Check sheet for the modelled part. Datum: model origin and axes. Units: mm. A direction names the side the tool comes from. Give positions to 0.01 mm unless a question says otherwise; leave off trailing zeros. Write each loop counter-clockwise with the first axis right and the second up, starting at its lowest first coordinate (ties: lowest second). Pieces come first, ordered by that corner, then holes. Notation, with made-up numbers: M 1,41 L 8,41 A19 ccw 8,68 Z; hole C 16.25,-24.75 d3. An arc over 180 degrees is marked long. Write item = value, one per line. Start each with the question number.
1) Cross-section at B-B, the plane x = -9. Record the cut outline in (y, z).
2) Go/stop test with flat-tipped pins: pin 1 (1.6 mm diameter, centred on x = 9, z = -0.5, fed in from -Y); pin 2 (2 mm diameter, centred on x = 10, z = 0, fed in from -Y); pin 3 (1.5 mm diameter, centred on x = -1, z = 2.5, fed in from +Y). Record where each tip stops, or that it passes through.
3) Mould release check, pull along X, two halves, no side actions. Record for faces 1 (the flat face through (0, -5, -4)), 2 (the flat face through (7.25, -6, 0)), 3 (the flat face through (-14, -4, 0)): released by +X, released by -X, zero draft, split by the parting line, or undercut.
4) Cross-section at D-D, the plane y = -2.75. Record the cut outline in (x, z).
5) Access from +Z, -Z, +X, -X, +Y, -Y to the whole of each face (thin tool, end or side, straight path). Record for faces 4 (the flat face through (11.394, -6.281, 2.37)), 5 (the flat face through (8, -0.5, 1)).
6) Cross-section at C-C, the plane y = -6.5. Record the cut outline in (x, z).
7) Cross-section at A-A, the plane z = 0. Give the number of separate pieces and of enclosed holes in the cut face, plus the area to 3 significant figures.
8) Scan lines: line 1 along X through (y, z) = (-5.5, -1); line 2 along Z through (x, y) = (10, -2.75); line 3 along X through (y, z) = (-3, 0.25). Record each from-to range of solid material in increasing order. Write a range as [from, to].
```python
from build123d import *

# Parameters (mm, degrees)
BOSS_EXTRUDE1_DEPTH  = 4
M3_CLEARANCE_HOLE1_D = 3.4
CUT_EXTRUDE1_DEPTH   = 3


with BuildPart() as part:
    # Sketch1 → Boss-Extrude1 (new, symmetric)
    with BuildSketch(Plane.XY):
        with BuildLine():
            Line((14, -0.5), (4.736180555, -0.5))
            ThreePointArc((4.736180555, -0.5), (0, -4.7625), (-4.736180555, -0.5))
            Line((-4.736180555, -0.5), (-14, -0.5))
            Line((-14, -0.5), (-14, -7.76))
            Line((-14, -7.76), (14, -7.76))
            Line((14, -7.76), (14, -0.5))
        make_face()
    extrude(amount=BOSS_EXTRUDE1_DEPTH, both=True)

    # M3 Clearance Hole1 (through all)
    with Locations(Plane.XZ.offset(7.76)):
        with Locations((-10, 0), (10, 0)):
            Hole(M3_CLEARANCE_HOLE1_D / 2)

    # Sketch5 → Cut-Extrude1 (cut)
    with BuildSketch(Plane.XZ.offset(7.76)):
        Polygon((-7.25, -1.58771324), (-7.25, 1.58771324), (-10, 3.175426481), (-12.75, 1.58771324), (-12.75, -1.58771324), (-10, -3.175426481), align=None)
        Polygon((7.25, -1.58771324), (10, -3.175426481), (12.75, -1.58771324), (12.75, 1.58771324), (10, 3.175426481), (7.25, 1.58771324), align=None)
    extrude(amount=-CUT_EXTRUDE1_DEPTH, mode=Mode.SUBTRACT)


solid = part.part
```
Reply:
q1.outline = M -7.76,-4 L -0.5,-4 L -0.5,-1.37 L -4.76,-1.37 L -4.76,-2.6 L -7.76,-2.6 Z; M -7.76,2.6 L -4.76,2.6 L -4.76,1.37 L -0.5,1.37 L -0.5,4 L -7.76,4 Z
q2.pin_1 = -4.76
q2.pin_2 = through
q2.pin_3 = -4.43
q3.face_1 = zero draft
q3.face_2 = undercut
q3.face_3 = released by -X
q4.outline = M -14,-4 L -3.89,-4 L -3.89,4 L -14,4 Z; M 3.89,-4 L 14,-4 L 14,4 L 3.89,4 Z; hole C -10,0 d3.4; hole C 10,0 d3.4
q5.face_4 = -Y
q5.face_5 = +Z, -Z, +X, -X, +Y
q6.outline = M -14,-4 L 14,-4 L 14,4 L -14,4 Z; hole M -12.75,-1.59 L -10,-3.18 L -7.25,-1.59 L -7.25,1.59 L -10,3.18 L -12.75,1.59 Z; hole M 7.25,-1.59 L 10,-3.18 L 12.75,-1.59 L 12.75,1.59 L 10,3.18 L 7.25,1.59 Z
q7.separate_pieces = 3
q7.enclosed_holes = 0
q7.area = 110 mm2
q8.line_1 = [-14, -12.75], [-7.25, 7.25], [12.75, 14]
q8.line_2 = [-4, -1.7], [1.7, 4]
q8.line_3 = [-14, -11.68], [-8.32, -3.7], [3.7, 8.32], [11.68, 14]
